Build history of the part. All positions in model axes, mm. Coordinates: 2 decimals unless noted, no trailing zeros. Loops run counter-clockwise (first coordinate to the right, second up) from the corner with the lowest first, then second, coordinate; pieces in that order, holes last.
(1) Slice it at A-A (y = 50.25). Give the cut face in (x, z).
(2) Slice it at B-B (z = 6.75). Give the cut face in (x, y), and give its area (3 significant figures).
(3) Flat gauge pins, fed straight in: P1, Ø4, axis at y = 44.5, z = 8.5, coming from the -X side; P2, Ø9.5, axis at x = 105.77, y = 42.89, coming from the -Z side; P3, Ø11, axis at x = 107, y = 39, coming from the +Z side; P4, Ø2.5, axis at y = 37.5, z = 7, coming from the +X side. Where does each tip first touch, or does it go through?
(4) Wall check: L1, parallel to X at y = 41.5, z = 3.5; L2, parallel to X at y = 38, z = 9.5; L3, parallel to Z at x = 99.5, y = 52.75. Give the ranges that are in metal, low to high.
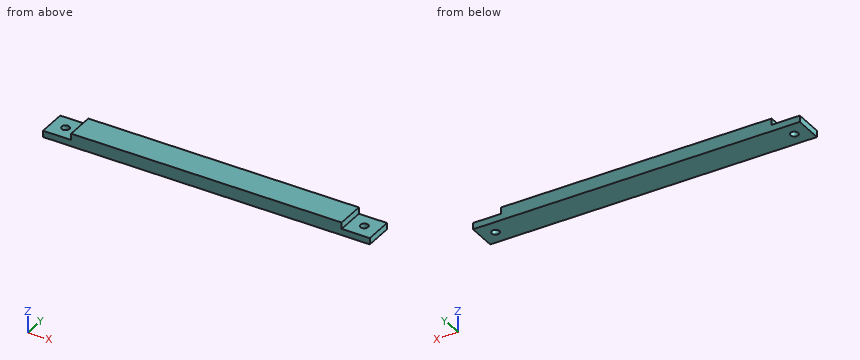
from build123d import *

# Parameters (mm, degrees)
ESQUISSE1_W             = 255.49
ESQUISSE1_H             = 22
ESQUISSE1_R             = 3
BOSS_EXTRU_1_DEPTH      = 10
ESQUISSE2_W             = 22
ESQUISSE2_H             = 22
ENL_V_MAT_EXTRU_1_DEPTH = 5


with BuildPart() as part:
    # Esquisse1 → Boss.-Extru.1 (new body)
    with BuildSketch(Plane.XY):
        with Locations((-10.977028198, 42.888888889)):
            Rectangle(ESQUISSE1_W, ESQUISSE1_H)
        with Locations((-127.722028198, 42.888888889)):
            Circle(ESQUISSE1_R, mode=Mode.SUBTRACT)
        with Locations((105.767971802, 42.888888889)):
            Circle(ESQUISSE1_R, mode=Mode.SUBTRACT)
    extrude(amount=BOSS_EXTRU_1_DEPTH)

    # Esquisse2 → Enlèv. mat.-Extru.1 (cut)
    with BuildSketch(Plane.XY.offset(10)):
        with Locations((-127.722028198, 42.888888889)):
            Rectangle(ESQUISSE2_W, ESQUISSE2_H)
        with Locations((105.767971802, 42.888888889)):
            Rectangle(ESQUISSE2_W, ESQUISSE2_H)
    extrude(amount=-ENL_V_MAT_EXTRU_1_DEPTH, mode=Mode.SUBTRACT)


solid = part.part
Response values:
1. outline: (-138.72, 0) - (116.77, 0) - (116.77, 5) - (94.77, 5) - (94.77, 10) - (-116.72, 10) - (-116.72, 5) - (-138.72, 5) - close
2. outline: (-116.72, 31.89) - (94.77, 31.89) - (94.77, 53.89) - (-116.72, 53.89) - close
2. area: 4,650 mm2
3. P1: stops at x = -116.72
3. P2: stops at z = 0
3. P3: stops at z = 5
3. P4: stops at x = 94.77
4. L1: x = -138.72 to -130.38, -125.06 to 103.11, 108.43 to 116.77
4. L2: x = -116.72 to 94.77
4. L3: z = 0 to 5
